Build history of the part. All positions in model axes, mm. A direction names the side the tool comes from. Round coordinates to 2 decimals unless told otherwise and drop trailing zeros. Loops run counter-clockwise (first coordinate to the right, second up) from the corner with the lowest first, then second, coordinate; pieces in that order, holes last. Notation, with made-up numbers: (-14, 87) - (-6, 87) arc R7 ccw to (-6, 98) - close; hole circle Ø3 at (27.5, 24). An arc over 180 degrees is marked (long way). Use a Markdown table: item, result.
from build123d import *

# Parameters (mm, degrees)
BOSS_EXTRUDE1_START = 0.25
SKETCH1_W           = 48.563793396
SKETCH1_H           = 23.003536126
SKETCH1_R           = 4.25
BOSS_EXTRUDE1_DEPTH = 3


with BuildPart() as part:
    # Sketch1 → Boss-Extrude1 (new body)
    with BuildSketch(Plane.XY.offset(75.780531955).offset(BOSS_EXTRUDE1_START)):
        with Locations((32.639628913, 33.325057501)):
            Rectangle(SKETCH1_W, SKETCH1_H)
        with Locations((18.660828036, 30.906825564)):
            Circle(SKETCH1_R, mode=Mode.SUBTRACT)
        with BuildLine():
            Line((37.818598421, 32.735851952), (37.818598421, 27.735851952))
            ThreePointArc((37.818598421, 27.735851952), (38.096846979, 27.06410051), (38.768598421, 26.785851952))
            Line((38.768598421, 26.785851952), (47.868598421, 26.785851952))
            ThreePointArc((47.868598421, 26.785851952), (48.540349863, 27.06410051), (48.818598421, 27.735851952))
            Line((48.818598421, 27.735851952), (48.818598421, 32.735851952))
            ThreePointArc((48.818598421, 32.735851952), (48.540349863, 33.407603394), (47.868598421, 33.685851952))
            Line((47.868598421, 33.685851952), (38.768598421, 33.685851952))
            ThreePointArc((38.768598421, 33.685851952), (38.096846979, 33.407603394), (37.818598421, 32.735851952))
        make_face(mode=Mode.SUBTRACT)
    extrude(amount=BOSS_EXTRUDE1_DEPTH)


solid = part.part
Q1. Cut at C-C, the plane x = 18. List the corners of the cut face in (y, z).
Results found:
| item | result |
|---|---|
| outline | (21.82, 76.03) - (26.71, 76.03) - (26.71, 79.03) - (21.82, 79.03) - close; (35.11, 76.03) - (44.83, 76.03) - (44.83, 79.03) - (35.11, 79.03) - close |
Q2. Which spindle directions (+Z, -Z, +X, -X, +Y, -Y) get a long thin tool onto all of the face, cutting with end or side? Do faces 4 (the face through (8.358, 33, 78)), 5 (the face through (43, 33.686, 78)). Say none if no direction does.
Results found:
| item | result |
|---|---|
| face 4 | +Z, -Z, -X, +Y, -Y |
| face 5 | +Z, -Z |
Q3. Pull direction Z, two halves, no side cores. Call faces 1 (the face through (32, 33, 76.031)), 2 (the face through (38.09, 27.07, 77.51)), 3 (the face through (32, 33, 79.031)): pulls with the +Z half, pulls with the -Z half, needs draft (parallel to the pull), parting line crosses it, or undercut.
Results found:
| item | result |
|---|---|
| face 1 | pulls with the -Z half |
| face 2 | needs draft |
| face 3 | pulls with the +Z half |
Q4. Cut at B-B, the plane z = 78.4. List the corners of the cut face in (x, y).
Results found:
| item | result |
|---|---|
| outline | (8.36, 21.82) - (56.92, 21.82) - (56.92, 44.83) - (8.36, 44.83) - close; hole circle Ø8.5 at (18.66, 30.91); hole (37.82, 27.74) arc R0.95 ccw to (38.77, 26.79) - (47.87, 26.79) arc R0.95 ccw to (48.82, 27.74) - (48.82, 32.74) arc R0.95 ccw to (47.87, 33.69) - (38.77, 33.69) arc R0.95 ccw to (37.82, 32.74) - close |
Q5. Probe line 1 (X direction, y = 31, z = 76.55); line 2 (Y direction, x = 41.5, z = 77.4); line 3 (X direction, y = 28, z = 76.8). List the from-to ranges inside material, lowest first.
Results found:
| item | result |
|---|---|
| line 1 | x = 8.36 to 14.41, 22.91 to 37.82, 48.82 to 56.92 |
| line 2 | y = 21.82 to 26.79, 33.69 to 44.83 |
| line 3 | x = 8.36 to 15.56, 21.76 to 37.82, 48.82 to 56.92 |
Q6. Drop a flat-ended pin along its axis: pin 1 (10 mm diameter, centred on x = 15.5, y = 32, fed in from -Z). Give the stop position or say it passes through.
Results found:
| item | result |
|---|---|
| pin 1 | stops at z = 76.03 |
Q7. Cut at A-A, the plane x = 43. List the corners of the cut face in (y, z).
Results found:
| item | result |
|---|---|
| outline | (21.82, 76.03) - (26.79, 76.03) - (26.79, 79.03) - (21.82, 79.03) - close; (33.69, 76.03) - (44.83, 76.03) - (44.83, 79.03) - (33.69, 79.03) - close |
